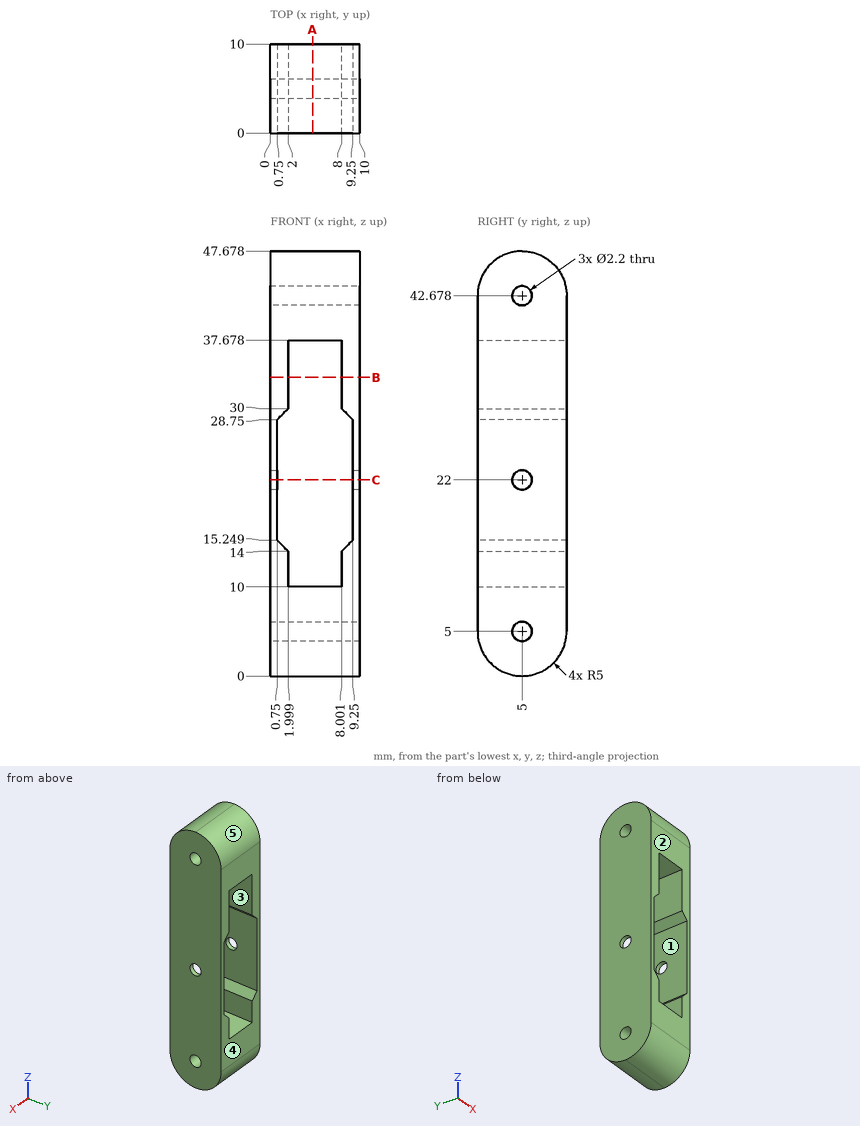
Here's the drawing with two shaded views (mm, measured from the low corner). I have some questions. A direction names the side the tool comes from. Coordinates: 2 decimals unless noted, no trailing zeros. Order: outer loops, then holes, each group sorted by start corner. A loop starts at its lowest first (then second) coordinate and runs counter-clockwise, first axis right, second up. Notation, with made-up numbers: (67.5, 49.25) - (117.5, 49.25) arc R22 ccw to (117.5, 73.25) - close; hole circle Ø10 at (9.5, -18). An arc over 180 degrees is marked (long way). Answer in a Markdown table with one row per item. Add a question column.
(1) If we mould it in two halves opening along Z, with no side actions, what happens to the marked faces 3, 4 and 5? For each: released by +Z, released by -Z, zero draft, split by the parting line, or undercut.
(2) On a 3-axis mill with a long thin cutter (end or side, diameter ignored), from which of +Z, -Z, +X, -X, +Y, -Y can I reach the whole of each face in a straight line? I mean the marked faces 1 and 2. Say none if no direction works.
(3) Will these pins go through, and if not, where does the flat tip stop? pin 1 (2.5 mm diameter, centred on y = 5, z = 42.678, fed in from -X); pin 2 (1.5 mm diameter, centred on x = 1, y = 3, fed in from +Z); pin 3 (2 mm diameter, centred on x = 3.5, y = 7, fed in from +Z).
(4) If we section it at A-A, the plane x = 4.75: State how many separate pieces and enclosed holes the cut face has, then the cut area to 3 significant figures.
(5) If we section it at B-B, the plane z = 33.5: Please give me the cut outline in (x, y), then the cut area to 3 significant figures.
(6) I need wall thicknesses on L1, parallel to Z at x = 9.4, y = 5; L2, parallel to Z at x = 5, y = 5; L3, parallel to X at y = 2.75, z = 33. Which ranges of each line are inside material? Lowest first, please.
(7) If we section it at C-C, the plane z = 22: Please give me the cut outline in (x, y).
Results are:
| question | item | result |
|---|---|---|
| 1 | face 3 | undercut |
| 1 | face 4 | zero draft |
| 1 | face 5 | released by +Z |
| 2 | face 1 | +Y, -Y |
| 2 | face 2 | +Z, -Z, +X, -X, -Y |
| 3 | pin 1 | stops at x = 0 |
| 3 | pin 2 | stops at z = 47.52 |
| 3 | pin 3 | stops at z = 47.58 |
| 4 | separate pieces | 2 |
| 4 | enclosed holes | 2 |
| 4 | area | 171 mm2 |
| 5 | outline | (0, 0) - (2, 0) - (2, 10) - (0, 10) - close; (8, 0) - (10, 0) - (10, 10) - (8, 10) - close |
| 5 | area | 40.0 mm2 |
| 6 | L1 | z = 0 to 3.9, 6.1 to 20.9, 23.1 to 41.58, 43.78 to 47.68 |
| 6 | L2 | z = 0 to 3.9, 6.1 to 10, 37.68 to 41.58, 43.78 to 47.68 |
| 6 | L3 | x = 0 to 2, 8 to 10 |
| 7 | outline | (0, 0) - (0.75, 0) - (0.75, 3.9) - (0, 3.9) - close; (0, 6.1) - (0.75, 6.1) - (0.75, 10) - (0, 10) - close; (9.25, 0) - (10, 0) - (10, 3.9) - (9.25, 3.9) - close; (9.25, 6.1) - (10, 6.1) - (10, 10) - (9.25, 10) - close |
